For this review, take the finished solid that the model builds, in its own axes (mm). A direction names the side the tool comes from. Coordinates: 2 decimals unless noted, no trailing zeros. Loops run counter-clockwise (first coordinate to the right, second up) from the corner with the lowest first, then second, coordinate; pieces in that order, holes last. Notation, with made-up numbers: (27.5, -39.75) -> (81.5, -39.75) arc R23 cw to (81.5, -30.75) -> close; hole circle Ø9 at (-26.5, -21). An arc over 180 degrees is marked (long way). One line per item, written item: value.
from build123d import *

# Parameters (mm, degrees)
SKETCH_R        = 1.8
SKETCH_W        = 41.028241
SKETCH_H        = 39
SKETCH_W_2      = 41
SKETCH_H_2      = 20.463
PAD_DEPTH       = 2
SKETCH001_R     = 3.8
SKETCH001_R_2   = 4
SKETCH001_R_3   = 1.8
PAD001_DEPTH    = 22
SKETCH002_R     = 8.25
POCKET_DEPTH    = 5
SKETCH003_R     = 1.8
POCKET001_DEPTH = 5
SKETCH004_W     = 53.310085
SKETCH004_H     = 13.854095
POCKET002_DEPTH = 5


with BuildPart() as part:
    # Sketch → Pad (new body)
    with BuildSketch(Plane.XY):
        Polygon((-53, 15), (53, 15), (53, -6.5), (88.355343, -41.855343), (55.105343, -75.105343), (20, -40), (-53, -40), align=None)
        with Locations((-49, 0)):
            Circle(SKETCH_R, mode=Mode.SUBTRACT)
        with Locations((39.3, 0)):
            Circle(SKETCH_R, mode=Mode.SUBTRACT)
        with Locations((13.2, -31.8)):
            Circle(SKETCH_R, mode=Mode.SUBTRACT)
        with Locations((13.2, -3.8)):
            Circle(SKETCH_R, mode=Mode.SUBTRACT)
        with Locations((-24.485879, -12.5)):
            Rectangle(SKETCH_W, SKETCH_H, mode=Mode.SUBTRACT)
        with Locations((24.528241, -16.768476)):
            Rectangle(SKETCH_W_2, SKETCH_H_2, mode=Mode.SUBTRACT)
        with BuildLine():
            ThreePointArc((-39.199998, -34.2), (-41, -36), (-39.199998, -37.8))
            Line((-39.199998, -37.8), (-36.200009, -37.8))
            ThreePointArc((-36.200009, -37.8), (-34.4, -36.000004), (-36.2, -34.2))
            Line((-39.199998, -34.2), (-36.2, -34.2))
        make_face(mode=Mode.SUBTRACT)
    extrude(amount=PAD_DEPTH)

    # Sketch001 → Pad001 (new body)
    with BuildSketch(Plane(origin=(0, 0, 0), x_dir=(1, 0, 0), z_dir=(0, 0, -1))):
        with Locations((0, 28)):
            Circle(SKETCH001_R)
        with Locations((-49, 0)):
            Circle(SKETCH001_R_2)
        with Locations((-49, 0)):
            Circle(SKETCH001_R_3, mode=Mode.SUBTRACT)
        with BuildLine():
            ThreePointArc((27.599984, 4), (23.6, -8e-06), (27.600001, -4))
            Line((27.600001, -4), (32.6, -4))
            ThreePointArc((32.6, -4), (36.6, 1e-05), (32.59998, 4))
            Line((27.599984, 4), (32.59998, 4))
        make_face()
        with BuildLine():
            ThreePointArc((27.599995, 1.85), (25.75, -3e-06), (27.600001, -1.85))
            Line((27.600001, -1.85), (32.6, -1.85))
            ThreePointArc((32.6, -1.85), (34.45, 4e-06), (32.599991, 1.85))
            Line((27.599995, 1.85), (32.599991, 1.85))
        make_face(mode=Mode.SUBTRACT)
    extrude(amount=PAD001_DEPTH)

    # Sketch002 → Pocket (cut)
    with BuildSketch(Plane.XY.offset(2)):
        with Locations((53.4328, -58.256155)):
            Circle(SKETCH002_R)
        with Locations((71.433789, -39.081839)):
            Circle(SKETCH002_R)
        with BuildLine():
            ThreePointArc((64.504552, -54.573607), (64.450253, -57.684403), (67.561049, -57.738702))
            Line((67.561049, -57.738702), (72.236758, -53.223423))
            ThreePointArc((72.236758, -53.223423), (72.291056, -50.112627), (69.18026, -50.058329))
            Line((64.504552, -54.573607), (69.18026, -50.058329))
        make_face()
    extrude(amount=-POCKET_DEPTH, mode=Mode.SUBTRACT)

    # Sketch003 → Pocket001 (cut)
    with BuildSketch(Plane.XY.offset(2)):
        with Locations((-38, 12)):
            Circle(SKETCH003_R)
    extrude(amount=-POCKET001_DEPTH, mode=Mode.SUBTRACT)

    # Sketch004 → Pocket002 (cut)
    with BuildSketch(Plane.XY.offset(2)):
        with Locations((30.683283, 10.927048)):
            Rectangle(SKETCH004_W, SKETCH004_H)
    extrude(amount=-POCKET002_DEPTH, mode=Mode.SUBTRACT)


solid = part.part
1. To check wall thickness, follow probe 1 along X at (y, z) = (0, -13.25); probe 2 along Y at (x, z) = (13.2, 1.2); probe 3 along Z at (x, y) = (45.5, -7). State the ranges of each line that lie inside material, in increasing order. Write a range as from..to.
Return value:
probe 1: x = -53..-50.8, -47.2..-45, 23.6..25.75, 34.45..36.6
probe 2: y = -40..-33.6, -30..-27, -6.54..-5.6, -2..4
probe 3: z = 0..2
2. Take a section at A-A, the plane z = -19.5. Give the boundary of the cut face in (x, y), and give its area (3 significant figures).
Return value:
outline: circle Ø8 at (-49, 0); circle Ø7.6 at (0, -28); (27.6, -4) -> (32.6, -4) arc R4 ccw to (32.6, 4) -> (27.6, 4) arc R4 ccw to start; hole circle Ø3.6 at (-49, 0); hole (27.6, -1.85) -> (32.6, -1.85) arc R1.85 ccw to (32.6, 1.85) -> (27.6, 1.85) arc R1.85 ccw to start
area: 146 mm2
3. Take a section at D-D, the plane x = 13.2. Give the boundary of the cut face in (y, z).
Return value:
outline: (-40, 0) -> (-33.6, 0) -> (-33.6, 2) -> (-40, 2) -> close; (-30, 0) -> (-27, 0) -> (-27, 2) -> (-30, 2) -> close; (-6.54, 0) -> (-5.6, 0) -> (-5.6, 2) -> (-6.54, 2) -> close; (-2, 0) -> (4, 0) -> (4, 2) -> (-2, 2) -> close
4. The part is to be moulded in two halves that separate along X. For faces 1 (the flat face through (71.96, -58.25, 0.99)), 2 (the cylindrical face through (69.645, -47.136, 1.014)), 3 (the flat face through (19, -29, 2)), say which applies: pulls with the +X half, pulls with the -X half, needs draft (parallel to the pull), parting line crosses it, or undercut.
Return value:
face 1: pulls with the +X half
face 2: undercut
face 3: needs draft
5. Take a section at C-C, the plane x = 39.3. Give the boundary of the cut face in (y, z), and give its area (3 significant figures).
Return value:
outline: (-59.3, 0) -> (-27, 0) -> (-27, 2) -> (-59.3, 2) -> close; (-6.54, 0) -> (-1.8, 0) -> (-1.8, 2) -> (-6.54, 2) -> close; (1.8, 0) -> (4, 0) -> (4, 2) -> (1.8, 2) -> close
area: 78.5 mm2
6. For faces 4 (the flat face through (0, -28, -22)), 5 (the flat face through (69.87, -55.51, 1.01)), 6 (the flat face through (30, -4, -11)), 7 (the flat face through (30, 1.85, -11)), 8 (the cylindrical face through (36.6, 0.1, -10.8)), list the 3-axis set-ups (+Z, -Z, +X, -X, +Y, -Y) from which the entire face can be reached by the end or side of a thin tool; tool diameter is ignored.
Return value:
face 4: -Z, +X, -X, +Y, -Y
face 5: +Z, -Z
face 6: -Z, +X, -X, -Y
face 7: -Z
face 8: -Z, +X
7. Take a section at B-B, the plane y = -15.5. Give the boundary of the cut face in (x, z).
Return value:
outline: (-53, 0) -> (-45, 0) -> (-45, 2) -> (-53, 2) -> close; (-3.97, 0) -> (4.03, 0) -> (4.03, 2) -> (-3.97, 2) -> close; (45.03, 0) -> (62, 0) -> (62, 2) -> (45.03, 2) -> close
8. Insertion check: pin 1 Ø2 at (y, z) = (-9, 0.5) entering from +X; pin 2 Ø0.6 at (x, z) = (-38, 1.5) entering from -Y; pin 3 Ø0.6 at (x, z) = (20.5, 1) entering from +Y. Each pin has a flat end and moves straight along its axis. Give the tip position at first contact, or say it passes through.
Return value:
pin 1: stops at x = 56.5
pin 2: stops at y = -40
pin 3: stops at y = 4
